```python
from build123d import *

# Parameters (mm, degrees)
SKETCH002_R      = 3.8
SKETCH002_R_2    = 1.8
PAD002_DEPTH     = 7
HOLE_D           = 4.4
HOLE_DEPTH       = 0.8
HOLE_CSINK_D     = 4.8
HOLE_CSINK_ANGLE = 90
HOLE_TIPS_R      = 2.2


with BuildPart() as part:
    # Sketch002 → Pad002 (new body)
    with BuildSketch(Plane.XY):
        Circle(SKETCH002_R)
        Circle(SKETCH002_R_2, mode=Mode.SUBTRACT)
    extrude(amount=-PAD002_DEPTH)

    # Hole
    with Locations(Plane.XY):
        with Locations((0, 0)):
            CounterSinkHole(HOLE_D / 2, HOLE_CSINK_D / 2, depth=HOLE_DEPTH, counter_sink_angle=HOLE_CSINK_ANGLE)

    # Hole tips → Hole tip 1 section 0
    with BuildSketch(Plane.XY.offset(-0.8), mode=Mode.PRIVATE) as hole_tip_1_s0:
        Circle(HOLE_TIPS_R)
    loft([hole_tip_1_s0.sketch, Vertex(0, 0, -2.121893)], mode=Mode.SUBTRACT)


solid = part.part
```
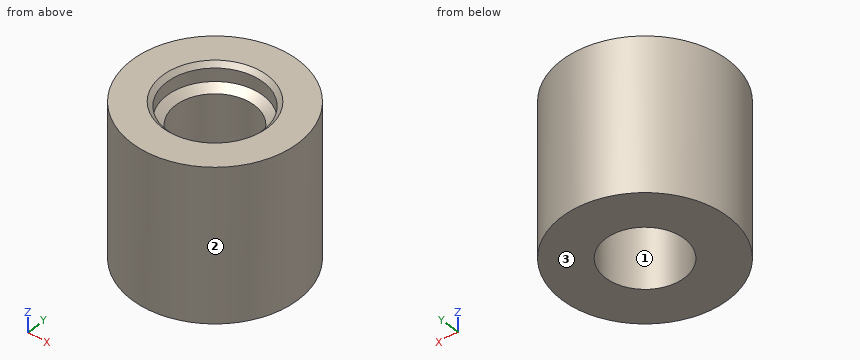
Check sheet for the modelled part. Datum: model origin and axes. Units: mm. Face numbers are marked on the shaded views. Coordinates: 2 decimals unless noted, no trailing zeros. Order: outer loops, then holes, each group sorted by start corner. A loop starts at its lowest first (then second) coordinate and runs counter-clockwise, first axis right, second up. Notation, with made-up numbers: (69.5, -33) -> (117.5, -33) arc R8 ccw to (117.5, -18) -> close; hole circle Ø7 at (1.25, -16.75). An arc over 180 degrees is marked (long way). Write each question's results on one line, items separated by ' | '. Start each with the question number.
1) Section check D-D (x = -3.5). Enter the section's corners in (y, z).
2) Material ranges on line 1 along Y through (x, z) = (0, -0.35); line 2 along X through (y, z) = (0.5, -1.5); line 3 along Y through (x, z) = (-1.25, -3.75), recorded low to high.
3) Section check A-A (x = 0). Enter the section's corners in (y, z), and give its area (3 significant figures).
4) Section check B-B (z = -2.75). Enter the section's corners in (x, y).
5) Section check C-C (y = -3). Enter the section's corners in (x, z), and give its area (3 significant figures).
6) Depth check by flat-ended pin: pin 1 (4 mm diameter, centred on x = 0, y = 0, fed in from +Z); pin 2 (1 mm diameter, centred on x = 2, z = -4, fed in from +Y); pin 3 (1 mm diameter, centred on y = -1.5, z = -5.5, fed in from -X). Enter the tip coordinate at first touch or a pass-through.
7) Draft check along X on the marked faces 1, 2 and 3. Enter one of: pulls with the +X half, pulls with the -X half, needs draft (parallel to the pull), parting line crosses it, or undercut.
Checked values:
1) outline: (-1.48, -7) -> (1.48, -7) -> (1.48, 0) -> (-1.48, 0) -> close
2) line 1: -3.8 to -2.2, 2.2 to 3.8 | line 2: -3.77 to -1.73, 1.73 to 3.77 | line 3: -3.59 to -1.3, 1.3 to 3.59
3) outline: (-3.8, -7) -> (-1.8, -7) -> (-1.8, -1.04) -> (-2.2, -0.8) -> (-2.2, -0.2) -> (-2.4, 0) -> (-3.8, 0) -> close; (1.8, -7) -> (3.8, -7) -> (3.8, 0) -> (2.4, 0) -> (2.2, -0.2) -> (2.2, -0.8) -> (1.8, -1.04) -> close | area: 27.2 mm²
4) outline: circle Ø7.6 at (0, 0); hole circle Ø3.6 at (0, 0)
5) outline: (-2.33, -7) -> (2.33, -7) -> (2.33, 0) -> (-2.33, 0) -> close | area: 32.7 mm²
6) pin 1: z = -0.92 | pin 2: y = 3.49 | pin 3: x = -3.67
7) face 1: undercut | face 2: parting line crosses it | face 3: needs draft
